```python
from build123d import *

# Parameters (mm, degrees)
SKETCH1_R           = 5.25
BOSS_EXTRUDE1_DEPTH = 19.5
BOSS_EXTRUDE2_DEPTH = 10.5
FILLET1_R           = 1
CUT_EXTRUDE1_DEPTH  = 0.6


with BuildPart() as part:
    # Sketch1 → Boss-Extrude1 (new, symmetric)
    with BuildSketch(Plane(origin=(0, 0, 0), x_dir=(0, 0, -1), z_dir=(1, 0, 0))):
        Circle(SKETCH1_R)
    extrude(amount=BOSS_EXTRUDE1_DEPTH, both=True)

    # Sketch2 → Boss-Extrude2 (add)
    with BuildSketch(Plane.XY.offset(5.25)):
        Polygon((-32.45, -8.15), (-11.6, -8.15), (-11.6, 0), (-11, 0), (-11, -8.75), (-32.45, -8.75), align=None)
        Polygon((32.45, -8.15), (11.6, -8.15), (11.6, 0), (11, 0), (11, -8.75), (32.45, -8.75), align=None)
    extrude(amount=-BOSS_EXTRUDE2_DEPTH)

    # Fillet1
    fillet1_edges = [part.edges().sort_by_distance(p)[0] for p in [
        (-11, -8.75, 0),
        (-11.6, -8.15, 0),
        (11.6, -8.15, 0),
        (11, -8.75, 0),
    ]]
    fillet(fillet1_edges, radius=FILLET1_R)

    # Sketch3 → Cut-Extrude1 (cut)
    with BuildSketch(Plane(origin=(0, -8.15, 0), x_dir=(1, 0, 0), z_dir=(0, 1, 0))):
        with BuildLine():
            Line((-24.95, -2.5), (-27.95, -2.5))
            ThreePointArc((-27.95, -2.5), (-30.45, 0), (-27.95, 2.5))
            Line((-27.95, 2.5), (-24.95, 2.5))
            ThreePointArc((-24.95, 2.5), (-22.45, 0), (-24.95, -2.5))
        make_face()
        with BuildLine():
            Line((24.95, -2.5), (27.95, -2.5))
            ThreePointArc((27.95, -2.5), (30.45, 0), (27.95, 2.5))
            Line((27.95, 2.5), (24.95, 2.5))
            ThreePointArc((24.95, 2.5), (22.45, 0), (24.95, -2.5))
        make_face()
    extrude(amount=-CUT_EXTRUDE1_DEPTH, mode=Mode.SUBTRACT)


solid = part.part
```
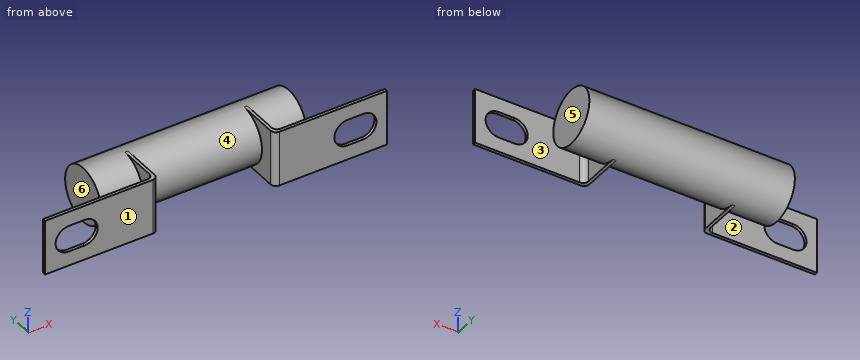
Source: CAD feature listing. Evaluate the final solid. Frame: model axes, mm. Face numbers are marked on the shaded views. A direction names the side the tool comes from. Round coordinates to 2 decimals unless told otherwise and drop trailing zeros. Write each loop counter-clockwise with the first axis right and the second up, starting at its lowest first coordinate (ties: lowest second). Pieces come first, ordered by that corner, then holes. Notation, with made-up numbers: M -9,69 L 23,69 A16 cw 23,85 Z; hole C 88.5,60.5 d1. An arc over 180 degrees is marked long. Use CSV: the item, a comma, the result in double quotes. Start each with the question number.
Q1. Cut plane C-C on z = -3.75. Output: boundary loops of the cut face in (x, y), plus the area to 3 significant figures.
Q2. Cut plane A-A on z = 0. Output: boundary loops of the cut face in (x, y), plus the area to 3 significant figures.
Q3. Cut plane D-D on x = -8. Output: boundary loops of the cut face in (y, z), plus the area to 3 significant figures.
Q4. Access query for the marked faces 1, 2 and 3. Directions: +Z, -Z, +X, -X, +Y, -Y. A direction counts if a zero-diameter tool reaches every point of the face in a straight line with its end or side. Return the directions, or none.
Q5. First-contact query: P1, Ø1.5, axis at x = 15.5, z = 2.5, coming from the +Y side; P2, Ø3, axis at y = 1.5, z = 2, coming from the -X side; P3, Ø6, axis at x = -24.5, y = -7.5, coming from the +Z side; P4, Ø3, axis at x = -26.5, z = 0, coming from the +Y side. Flat tips, straight axial feed; report the tip coordinate or a pass-through.
Q6. Pull-direction query (X, two-part tool) for the marked faces 4, 5 and 6; classes: +X half, -X half, draft (parallel to the pull), parting line (faces both ways), or undercut.
Q7. Cut plane B-B on y = -4.5. Output: boundary loops of the cut face in (x, z).
Q8. Line query: line 1 (X direction, y = 1.5, z = 1.5); line 2 (Y direction, x = -14, z = 4.5); line 3 (X direction, y = -6.75, z = -4.75). Output: solid intervals per line, ascending. Write a range as from..to.
Results found:
1,outline,"M -32.45,-8.75 L -12,-8.75 A1 ccw -11,-7.75 L -11,-3.67 L 11,-3.67 L 11,-7.75 A1 ccw 12,-8.75 L 32.45,-8.75 L 32.45,-8.15 L 12.6,-8.15 A1 cw 11.6,-7.15 L 11.6,-3.67 L 19.5,-3.67 L 19.5,3.67 L -19.5,3.67 L -19.5,-3.67 L -11.6,-3.67 L -11.6,-7.15 A1 cw -12.6,-8.15 L -32.45,-8.15 Z"
1,area,"318 mm^2"
2,outline,"M -32.45,-8.75 L -30.45,-8.75 L -30.45,-8.15 L -32.45,-8.15 Z; M -22.45,-8.75 L -12,-8.75 A1 ccw -11,-7.75 L -11,-5.25 L 11,-5.25 L 11,-7.75 A1 ccw 12,-8.75 L 22.45,-8.75 L 22.45,-8.15 L 12.6,-8.15 A1 cw 11.6,-7.15 L 11.6,-5.25 L 19.5,-5.25 L 19.5,5.25 L -19.5,5.25 L -19.5,-5.25 L -11.6,-5.25 L -11.6,-7.15 A1 cw -12.6,-8.15 L -22.45,-8.15 Z; M 30.45,-8.75 L 32.45,-8.75 L 32.45,-8.15 L 30.45,-8.15 Z"
2,area,"429 mm^2"
3,outline,"C 0,0 d10.5"
3,area,"86.6 mm^2"
4,face 1,"+Z, -Z, +X, -X, -Y"
4,face 2,"+Z, -Z, -X"
4,face 3,"+Z, -Z, +X"
5,P1,"y = 4.95"
5,P2,"x = -19.5"
5,P3,"z = 5.25"
5,P4,"through"
6,face 4,"undercut"
6,face 5,"+X half"
6,face 6,"-X half"
7,outline,"M -19.5,-2.7 L -11.6,-2.7 L -11.6,-5.25 L -11,-5.25 L -11,-2.7 L 11,-2.7 L 11,-5.25 L 11.6,-5.25 L 11.6,-2.7 L 19.5,-2.7 L 19.5,2.7 L 11.6,2.7 L 11.6,5.25 L 11,5.25 L 11,2.7 L -11,2.7 L -11,5.25 L -11.6,5.25 L -11.6,2.7 L -19.5,2.7 Z"
8,line 1,"-19.5..19.5"
8,line 2,"-8.75..-8.15, -2.7..2.7"
8,line 3,"-11.6..-11, 11..11.6"
